Verification items for the finished model (mm, model axes). Face numbers are marked on the shaded views. A direction names the side the tool comes from. Coordinates: 2 decimals unless noted, no trailing zeros. Order: outer loops, then holes, each group sorted by start corner. A loop starts at its lowest first (then second) coordinate and runs counter-clockwise, first axis right, second up. Notation, with made-up numbers: M -29.75,-31 L 8.25,-31 A28 ccw 8.25,-6 Z; hole C 16.25,55 d3. An arc over 180 degrees is marked long. Return JSON: item names as keys, results as strings. Group by question number.
1. Material ranges on line 1 along X through (y, z) = (-16, 14); line 2 along X through (y, z) = (-25, 14.25); line 3 along Y through (x, z) = (-4, 2.25), recorded low to high.
2. Set-up check for the marked faces 1, 2 and 3: record each of +Z, -Z, +X, -X, +Y, -Y from which the full face is reachable in a straight line by a thin tool's end or side.
3. Gauge pin test, flat ends, axial feed: pin 1 (10 mm diameter, centred on y = 17.5, z = 11.5, fed in from -X); pin 2 (8 mm diameter, centred on y = -12.5, z = 7.5, fed in from -X); pin 3 (1.5 mm diameter, centred on x = 25, z = 11.5, fed in from +Y); pin 4 (12 mm diameter, centred on x = -12, y = -4.5, fed in from +Z). Record the tip position at first contact, or that the pin passes through.
4. Section check B-B, the plane x = 25.5. Record the cut outline in (y, z), plus the area to 3 significant figures.
5. Section check A-A, the plane y = -26.5. Record the cut outline in (x, z), plus the area to 3 significant figures.
6. Section check C-C, the plane z = 16.5. Record the cut outline in (x, y), plus the area to 3 significant figures.
7. Mould release check, pull along X, two halves, no side actions. Record for the marked faces 4, 5, 6 and 7: +X half, -X half, draft (parallel to the pull), parting line (faces both ways), or undercut.
8. Section check D-D, the plane y = 0. Record the cut outline in (x, z), plus the area to 3 significant figures.
Autodesk Fusion 360 part; units mm, degrees
sketch "Sketch1" plane through (0, 0, 0) normal (0, 0, 1) x (1, 0, 0)
  line L0 (0.7071, 27.5772) -> (23.2843, 5)
  line L1 (23.2843, -5) -> (0.7071, -27.5772)
  line L2 (-0.7071, -27.5772) -> (-25.2843, -3)
  line L3 (-25.2843, 3) -> (-0.7071, 27.5772)
  line L4 (0, 0) -> (57.5603, 0) construction
  line L5 (31, 0) -> (31, -17.1775)
  line L6 (-25.2843, 3) -> (-30.8545, 3)
  line L7 (-25.2843, -3) -> (-30.8545, -3)
  arc A0 (0.7071, 27.5772) -> (-0.7071, 27.5772) centre (0, 26.8701) ccw
  arc A1 (-0.7071, -27.5772) -> (0.7071, -27.5772) centre (0, -26.8701) ccw
  arc A2 (-30.8545, -3) -> (-30.8545, 3) centre (0, 0) ccw
  line L8 (26.2897, 5) -> (23.2843, 5)
  line L9 (26.2897, -5) -> (23.2843, -5)
  arc A3 (28.2701, -3.2791) -> (28.2701, 3.2791) centre (5, 0) ccw
  arc A4 (28.2701, 3.2791) -> (26.2897, 5) centre (26.2897, 3) ccw
  arc A5 (26.2897, -5) -> (28.2701, -3.2791) centre (26.2897, -3) ccw
  point P0 (0, 28.2843)
  point P1 (28.2843, 0)
  point P2 (29, 5)
  dimension "d1" = 62
  dimension "d2" = 40
  dimension "d4" = 20
  dimension "d5" = 20
  dimension "d7" = 45
  dimension "d9" = 3
  dimension "d11" = 1
  dimension "d13" = 5
  dimension "d14" = 5
  dimension "d15" = 47
  dimension "d16" = 2
extrude "Extrude1" add sketch "Sketch1" along normal blind 20
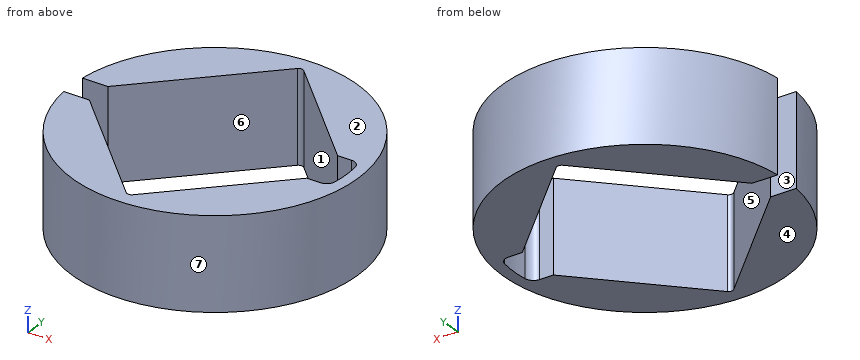
Answers follow:
{
 "1": {"line 1": "-26.55 to -12.28, 12.28 to 26.55", "line 2": "-18.33 to -3.28, 3.28 to 18.33", "line 3": "-30.74 to -24.28, 24.28 to 30.74"},
 "2": {"face 1": "+Z, -Z", "face 2": "+Z, +X, -X, +Y, -Y", "face 3": "+Z, -Z, -X"},
 "3": {"pin 1": "x = -28.37", "pin 2": "x = -29.81", "pin 3": "y = 19.31", "pin 4": "through"},
 "4": {"outline": "M -17.63,0 L -5,0 L -5,20 L -17.63,20 Z; M 5,0 L 17.63,0 L 17.63,20 L 5,20 Z", "area": "505 mm^2"},
 "5": {"outline": "M -16.09,0 L -1.78,0 L -1.78,20 L -16.09,20 Z; M 1.78,0 L 16.09,0 L 16.09,20 L 1.78,20 Z", "area": "572 mm^2"},
 "6": {"outline": "M -30.85,-3 A31 ccw long -30.85,3 L -25.28,3 L -0.71,27.58 A1 cw 0.71,27.58 L 23.28,5 L 26.29,5 A2 cw 28.27,3.28 A23.5 cw 28.27,-3.28 A2 cw 26.29,-5 L 23.28,-5 L 0.71,-27.58 A1 cw -0.71,-27.58 L -25.28,-3 Z", "area": "1,370 mm^2"},
 "7": {"face 4": "draft", "face 5": "undercut", "face 6": "undercut", "face 7": "parting line"},
 "8": {"outline": "M 28.5,0 L 31,0 L 31,20 L 28.5,20 Z", "area": "50.0 mm^2"}
}
